Read the model definition and answer for the solid it produces. Units are mm, in the model's axes. A direction names the side the tool comes from. Give positions to 0.01 mm unless a question says otherwise; leave off trailing zeros. Write each loop counter-clockwise with the first axis right and the second up, starting at its lowest first coordinate (ties: lowest second). Pieces come first, ordered by that corner, then holes. Notation, with made-up numbers: (-23.75, -4.75) - (-0.75, -4.75) arc R35 ccw to (-0.75, 27.25) - close; hole circle Ø10 at (5, 48). An arc over 180 degrees is marked (long way). Answer as CSV lines item,"result".
```python
from build123d import *

# Parameters (mm, degrees)
SKETCH_W        = 58
SKETCH_H        = 29.6
PAD_DEPTH       = 1.5
SKETCH001_W     = 54
SKETCH001_H     = 26.2
PAD001_DEPTH    = 1.4
SKETCH002_W     = 52
SKETCH002_H     = 24.2
POCKET_DEPTH    = 1
SKETCH003_R     = 7.97
SKETCH003_R_2   = 1.06
SKETCH003_W     = 3
SKETCH003_H     = 6.5
POCKET001_DEPTH = 5


with BuildPart() as part:
    # Sketch → Pad (new body)
    with BuildSketch(Plane.XY):
        with Locations((29, 14.8)):
            Rectangle(SKETCH_W, SKETCH_H)
    extrude(amount=PAD_DEPTH)

    # Sketch001 (on Face6 of Pad) → Pad001 (join)
    with BuildSketch(Plane.XY.offset(1.5)):
        with Locations((29, 14.8)):
            Rectangle(SKETCH001_W, SKETCH001_H)
    extrude(amount=PAD001_DEPTH)

    # Sketch002 (on Face4 of Pad001) → Pocket (cut)
    with BuildSketch(Plane(origin=(0, 0, 0), x_dir=(1, 0, 0), z_dir=(0, 0, -1))):
        with Locations((29, -14.8)):
            Rectangle(SKETCH002_W, SKETCH002_H)
    extrude(amount=-POCKET_DEPTH, mode=Mode.SUBTRACT)

    # Sketch003 (on Face16 of Pocket) → Pocket001 (cut)
    with BuildSketch(Plane.XY.offset(2.9)):
        with Locations((16.33, 14.8)):
            Circle(SKETCH003_R)
        with Locations((41.67, 14.8)):
            Circle(SKETCH003_R)
        with Locations((29, 22.3)):
            Circle(SKETCH003_R_2)
        with Locations((29, 7.3)):
            Circle(SKETCH003_R_2)
        with Locations((29, 14.8)):
            Rectangle(SKETCH003_W, SKETCH003_H)
    extrude(amount=-POCKET001_DEPTH, mode=Mode.SUBTRACT)


solid = part.part
```
(1) For faces 4 (the flat face through (2, 15, 2)), 5 (the flat face through (27.5, 15, 2)), 6 (the flat face through (0, 15, 1)), 7 (the flat face through (29, 29.6, 1)), 8 (the flat face through (29, 9, 1)), determine the directions among +Z, -Z, +X, -X, +Y, -Y from which every point of the face is accessible in a straight line to the end or side of a thin tool.
Worked out:
face 4,"+Z, -X, +Y, -Y"
face 5,"+Z, -Z"
face 6,"+Z, -Z, -X, +Y, -Y"
face 7,"+Z, -Z, +X, -X, +Y"
face 8,"-Z"
(2) A cutting plane is placed at D-D (y = 24). Write down the section's boundary in (x, z).
Worked out:
outline,"(0, 0) - (3, 0) - (3, 1) - (55, 1) - (55, 0) - (58, 0) - (58, 1.5) - (56, 1.5) - (56, 2.9) - (2, 2.9) - (2, 1.5) - (0, 1.5) - close"
(3) Each of these flat-tipped pins is pushed along its axis until it touches: P1, Ø1.9, axis at x = 29, y = 22.3, coming from the +Z side; P2, Ø6, axis at x = 47, y = 18.5, coming from the +Z side; P3, Ø0.7, axis at y = 16, z = 2, coming from the +X side; P4, Ø0.6, axis at x = 29.5, z = 2, coming from the +Y side. Where does it stop, or does it pass through?
Worked out:
P1,"passes through"
P2,"stops at z = 2.9"
P3,"stops at x = 56"
P4,"stops at y = 27.9"
(4) A cutting plane is placed at B-B (y = 14.8). Write down the section's boundary in (x, z), and give its area (3 significant figures).
Worked out:
outline,"(0, 0) - (3, 0) - (3, 1) - (8.36, 1) - (8.36, 2.9) - (2, 2.9) - (2, 1.5) - (0, 1.5) - close; (24.3, 1) - (27.5, 1) - (27.5, 2.9) - (24.3, 2.9) - close; (30.5, 1) - (33.7, 1) - (33.7, 2.9) - (30.5, 2.9) - close; (49.64, 1) - (55, 1) - (55, 0) - (58, 0) - (58, 1.5) - (56, 1.5) - (56, 2.9) - (49.64, 2.9) - close"
area,"44.3 mm^2"
(5) A cutting plane is placed at A-A (x = 41.67). Write down the section's boundary in (y, z), and give its area (3 significant figures).
Worked out:
outline,"(0, 0) - (2.7, 0) - (2.7, 1) - (6.83, 1) - (6.83, 2.9) - (1.7, 2.9) - (1.7, 1.5) - (0, 1.5) - close; (22.77, 1) - (26.9, 1) - (26.9, 0) - (29.6, 0) - (29.6, 1.5) - (27.9, 1.5) - (27.9, 2.9) - (22.77, 2.9) - close"
area,"26.6 mm^2"
(6) Find the intervals of material crossed by L1, parallel to Y at x = 29, z = 2.3; L2, parallel to X at y = 14.75, z = 2.5; L3, parallel to X at y = 10.25, z = 0.75, in increasing order.
Worked out:
L1,"y = 1.7 to 6.24, 8.36 to 11.55, 18.05 to 21.24, 23.36 to 27.9"
L2,"x = 2 to 8.36, 24.3 to 27.5, 30.5 to 33.7, 49.64 to 56"
L3,"x = 0 to 3, 55 to 58"
(7) The mould has two halves that part along Y. Classify faces 1 (the flat face through (29, 18.05, 2)), 2 (the flat face through (29, 27.9, 2)), 3 (the flat face through (56, 15, 2)): +Y half, -Y half, draft (parallel to the pull), parting line (faces both ways), or undercut.
Worked out:
face 1,"undercut"
face 2,"+Y half"
face 3,"draft"
(8) A cutting plane is placed at C-C (x = 29). Write down the section's boundary in (y, z), and give its area (3 significant figures).
Worked out:
outline,"(0, 0) - (2.7, 0) - (2.7, 1) - (6.24, 1) - (6.24, 2.9) - (1.7, 2.9) - (1.7, 1.5) - (0, 1.5) - close; (8.36, 1) - (11.55, 1) - (11.55, 2.9) - (8.36, 2.9) - close; (18.05, 1) - (21.24, 1) - (21.24, 2.9) - (18.05, 2.9) - close; (23.36, 1) - (26.9, 1) - (26.9, 0) - (29.6, 0) - (29.6, 1.5) - (27.9, 1.5) - (27.9, 2.9) - (23.36, 2.9) - close"
area,"36.5 mm^2"
